Check sheet for the modelled part. Datum: model origin and axes. Units: mm. Face numbers are marked on the shaded views. A direction names the side the tool comes from. Round coordinates to 2 decimals unless told otherwise and drop trailing zeros. Order: outer loops, then holes, each group sorted by start corner. A loop starts at its lowest first (then second) coordinate and runs counter-clockwise, first axis right, second up.
```python
from build123d import *

# Parameters (mm, degrees)
BOSS_EXTRUDE1_DEPTH = 5
SKETCH2_W           = 22
SKETCH2_H           = 4
BOSS_EXTRUDE2_DEPTH = 30
BOSS_EXTRUDE3_START = -10.723792
BOSS_EXTRUDE3_DEPTH = 3
BOSS_EXTRUDE4_START = 11.276208
BOSS_EXTRUDE4_DEPTH = 3
FILLET1_R           = 3


with BuildPart() as part:
    # Sketch1 → Boss-Extrude1 (new body)
    with BuildSketch(Plane(origin=(0, 0, 0), x_dir=(1, 0, 0), z_dir=(0, 1, 0))):
        Polygon((0.27620797, 14.279620853), (11.27620797, 14.279620853), (11.27620797, -35.310215712), (-10.72379203, -35.310215712), (-10.72379203, 14.279620853), align=None)
        with BuildLine():
            Line((-4.048192251, -4.720379147), (-4.048192251, 3.279620853))
            ThreePointArc((-4.048192251, 3.279620853), (-0.048192251, 7.279620853), (3.951807749, 3.279620853))
            Line((3.951807749, 3.279620853), (3.951807749, -4.720379147))
            ThreePointArc((3.951807749, -4.720379147), (-0.048192251, -8.720379147), (-4.048192251, -4.720379147))
        make_face(mode=Mode.SUBTRACT)
        with BuildLine():
            Line((-4.048192251, -26.720379147), (-4.048192251, -18.720379147))
            ThreePointArc((-4.048192251, -18.720379147), (-0.048192251, -14.720379147), (3.951807749, -18.720379147))
            Line((3.951807749, -18.720379147), (3.951807749, -26.720379147))
            ThreePointArc((3.951807749, -26.720379147), (-0.048192251, -30.720379147), (-4.048192251, -26.720379147))
        make_face(mode=Mode.SUBTRACT)
    extrude(amount=BOSS_EXTRUDE1_DEPTH)

    # Sketch2 → Boss-Extrude2 (add)
    with BuildSketch(Plane(origin=(0, 0, 0), x_dir=(1, 0, 0), z_dir=(0, 1, 0))):
        with Locations((0.27620797, 12.279620853)):
            Rectangle(SKETCH2_W, SKETCH2_H)
    extrude(amount=BOSS_EXTRUDE2_DEPTH)

    # Sketch6 → Boss-Extrude3 (add)
    with BuildSketch(Plane(origin=(0, 0, 0), x_dir=(0, 0, -1), z_dir=(1, 0, 0)).offset(BOSS_EXTRUDE3_START)):
        Polygon((10.279620853, 30), (10.279620853, 5), (-14.720379147, 5), align=None)
    extrude(amount=BOSS_EXTRUDE3_DEPTH)

    # Sketch6<2> → Boss-Extrude4 (add)
    with BuildSketch(Plane(origin=(0, 0, 0), x_dir=(0, 0, -1), z_dir=(1, 0, 0)).offset(BOSS_EXTRUDE4_START)):
        Polygon((10.279620853, 30), (10.279620853, 5), (-14.720379147, 5), align=None)
    extrude(amount=-BOSS_EXTRUDE4_DEPTH)

    # Fillet1
    fillet1_edges = [part.edges().sort_by_distance(p)[0] for p in [
        (11.27620797, 2.5, 35.310215712),
        (-10.72379203, 2.5, 35.310215712),
    ]]
    fillet(fillet1_edges, radius=FILLET1_R)


solid = part.part
```
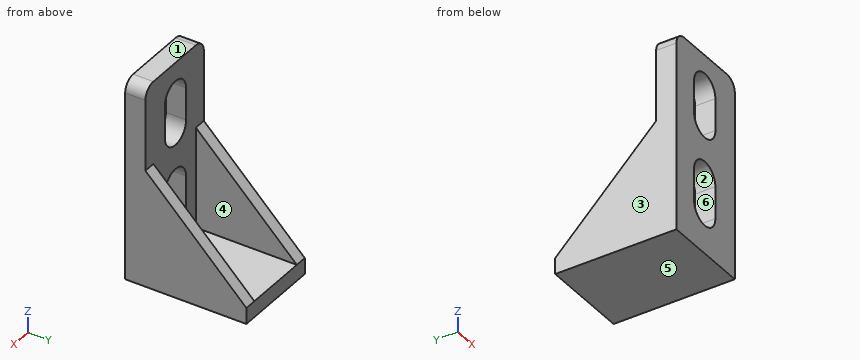
Item 1: Sectioned sample at A-A (z = 26). Record the cut outline in (x, y).
Answer:
outline: (-10.72, 0) - (-4.05, 0) - (-4.05, 5) - (-10.72, 5) - close; (3.95, 0) - (11.28, 0) - (11.28, 5) - (3.95, 5) - close
Item 2: Scan lines: line 1 along X through (y, z) = (10, -7); line 2 along Z through (x, y) = (2.75, 2); line 3 along Z through (x, y) = (6, 18). Record each from-to range of solid material in increasing order.
Answer:
line 1: x = -10.72 to -7.72, 8.28 to 11.28
line 2: z = -14.28 to -6.14, 7.58 to 15.86, 29.58 to 35.31
line 3: z = -14.28 to -10.28
Item 3: Access from +Z, -Z, +X, -X, +Y, -Y to the whole of each face (thin tool, end or side, straight path). Record for the marked faces 4, 5 and 6.
Answer:
face 4: +Z, +Y
face 5: -Z, +X, -X, +Y, -Y
face 6: +Y, -Y
Item 4: Sectioned sample at C-C (x = -3). Record the cut outline in (y, z), and give its area (3 significant figures).
Answer:
outline: (0, -14.28) - (30, -14.28) - (30, -10.28) - (5, -10.28) - (5, -5.98) - (0, -5.98) - close; (0, 7.42) - (5, 7.42) - (5, 16.02) - (0, 16.02) - close; (0, 29.42) - (5, 29.42) - (5, 35.31) - (0, 35.31) - close
area: 214 mm2
Item 5: Release check for a two-part mould opening along X. For the marked faces 1, 2 and 3 record: released by +X, released by -X, zero draft, split by the parting line, or undercut.
Answer:
face 1: zero draft
face 2: undercut
face 3: released by -X
Item 6: Sectioned sample at B-B (y = 4). Record the cut outline in (x, z), and give its area (3 significant figures).
Answer:
outline: (-10.72, -14.28) - (11.28, -14.28) - (11.28, 32.31) arc R3 ccw to (8.28, 35.31) - (-7.72, 35.31) arc R3 ccw to (-10.72, 32.31) - close; hole (-4.05, -3.28) arc R4 ccw to (3.95, -3.28) - (3.95, 4.72) arc R4 ccw to (-4.05, 4.72) - close; hole (-4.05, 18.72) arc R4 ccw to (3.95, 18.72) - (3.95, 26.72) arc R4 ccw to (-4.05, 26.72) - close
area: 859 mm2
Item 7: Go/stop test with flat-tipped pins: P1, Ø6, axis at x = -6, z = 27.5, coming from the -Y side; P2, Ø6, axis at x = -6.5, y = 18.5, coming from the +Z side; P3, Ø8, axis at x = 0, y = 18, coming from the +Z side; P4, Ø4, axis at x = -2, z = 28, coming from the +Y side. Record where each tip stops, or that it passes through.
Answer:
P1: stops at y = 0
P2: stops at z = 3.96
P3: stops at z = -10.28
P4: stops at y = 5
Item 8: Sectioned sample at D-D (y = 9.5). Record the cut outline in (x, z).
Answer:
outline: (-10.72, -14.28) - (11.28, -14.28) - (11.28, 10.22) - (8.28, 10.22) - (8.28, -10.28) - (-7.72, -10.28) - (-7.72, 10.22) - (-10.72, 10.22) - close
